Solid Edge part; units mm, degrees
sketch "Sketch1" plane through (0, 0, 44) normal (0, 0, 1) x (1, 0, 0)
  line L0 (33.1543, -1.1543) -> (24.7755, -1.1543)
  line L1 (24.7755, -1.1543) -> (24.7403, 8.3152)
  line L2 (24.7403, 8.3152) -> (33.048, 8.3152)
  line L3 (33.048, 8.3152) -> (33.048, 39.2077)
  line L4 (33.048, 39.2077) -> (54.894, 39.2077)
  line L5 (54.894, 39.2077) -> (54.894, 47.5424)
  line L6 (54.894, 47.5424) -> (64.0113, 47.5424)
  line L7 (64.0113, 47.5424) -> (64.1902, 47.5424)
  line L8 (64.1902, 47.5424) -> (64.1902, 39.2048)
  line L9 (64.1902, 39.2048) -> (104.7872, 39.2048)
  line L10 (104.7872, 39.2048) -> (104.7872, 47.5447)
  line L11 (104.7872, 47.5447) -> (114.1885, 47.5447)
  line L12 (114.1885, 47.5447) -> (114.1885, 39.2022)
  line L13 (114.1885, 39.2022) -> (137.8474, 39.2022)
  line L14 (137.8474, 39.2022) -> (137.8474, -32.2815)
  line L15 (137.8474, -32.2815) -> (114.1885, -32.2815)
  line L16 (114.1885, -32.2815) -> (114.1885, -40.4625)
  line L17 (114.1885, -40.4625) -> (104.7872, -40.4625)
  line L18 (104.7872, -40.4625) -> (104.7872, -32.2809)
  line L19 (104.7872, -32.2809) -> (64.2772, -32.2809)
  line L20 (64.2772, -32.2809) -> (64.2772, -40.4663)
  line L21 (64.2772, -40.4663) -> (54.6991, -40.4663)
  line L22 (54.6991, -40.4663) -> (54.6991, -32.2809)
  line L23 (54.6991, -32.2809) -> (33.1543, -32.2809)
  line L24 (33.1543, -32.2809) -> (33.1543, -1.1543)
extrude "Protrusion1" add sketch "Sketch1" along normal blind 4
hole "Hole_1" at (59.4881, -36.3736, 48) direction (0, 0, -1) diameter 3.4 end up to next
hole "Hole1" at (109.4878, -36.3718, 48) direction (0, 0, -1) diameter 3.4 end up to next
hole "Hole2" at (59.5729, 43.4608, 48) direction (0, 0, -1) diameter 3.4 end up to next
hole "Hole3" at (109.5725, 43.3528, 48) direction (0, 0, -1) diameter 3.4 end up to next
hole "Hole4" at (28.9649, 3.5805, 48) direction (0, 0, -1) diameter 3.4 end up to next
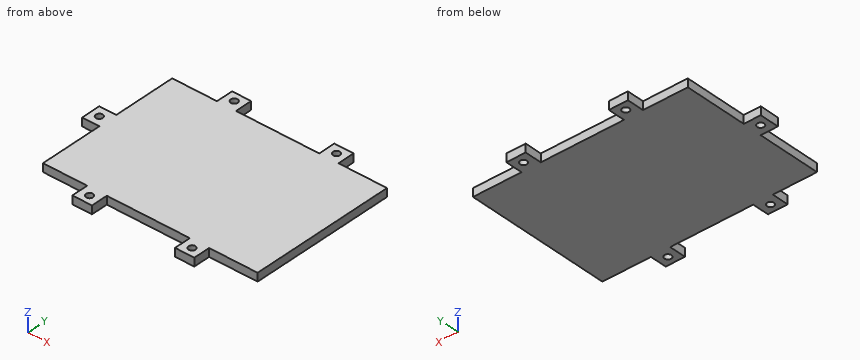
Source: CAD feature listing. Evaluate the final solid. Frame: model axes, mm. Give positions to 0.01 mm unless a question says otherwise; leave off trailing zeros. Write each loop counter-clockwise with the first axis right and the second up, starting at its lowest first coordinate (ties: lowest second). Pieces come first, ordered by that corner, then holes. Notation, with made-up numbers: (6, -32.75) - (25, -32.75) arc R22 ccw to (25, -21.75) - close; hole circle Ø6 at (84, -33.5). An arc over 180 degrees is marked (long way). Write item = value, one per line. Start each with the question number.
Q1. Cut plane B-B, the plane x = 117. Return loops of the section in (y, z), then the cut area to 3 significant figures.
Q2. Cut plane A-A, the plane z = 45.55. Give the number of separate pieces and of enclosed holes in the cut face, then the cut area to 3 significant figures.
Q3. Material intervals for probe 1 along Y at (x, z) = (59.5, 47.35); probe 2 along X at (y, z) = (-34, 45.9); probe 3 along Y at (x, z) = (110, 47.1), sorted ascending.
Q4. Pin query (flat end, axial travel): pin 1 Ø2 at (x, z) = (57, 45) entering from +Y; pin 2 Ø2.5 at (x, y) = (109.57, 43.35) entering from +Z; pin 3 Ø1.2 at (x, z) = (110, 47) entering from -Y; pin 4 Ø2 at (y, z) = (-37.5, 46.5) entering from -X. Return the tip coordinate at first contact, or that it passes through.
Q5. Cut plane C-C, the plane y = 12.5. Return loops of the section in (x, z).
Computed values:
q1.outline = (-32.28, 44) - (39.2, 44) - (39.2, 48) - (-32.28, 48) - close
q1.area = 286 mm²
q2.separate_pieces = 1
q2.enclosed_holes = 5
q2.area = 7,830 mm²
q3.probe_1 = -40.47 to -38.07, -34.67 to 41.76, 45.16 to 47.54
q3.probe_2 = 54.7 to 64.28, 104.79 to 114.19
q3.probe_3 = -40.46 to -37.99, -34.75 to 41.71, 45 to 47.54
q4.pin_1 = 47.54
q4.pin_2 = through
q4.pin_3 = -40.46
q4.pin_4 = 54.7
q5.outline = (33.05, 44) - (137.85, 44) - (137.85, 48) - (33.05, 48) - close
